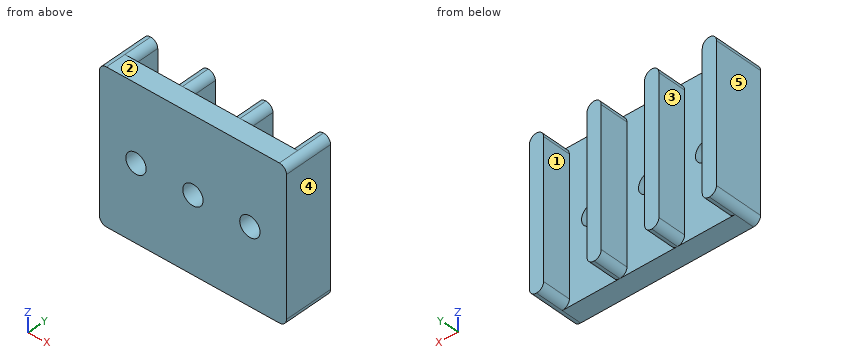
from build123d import *

# Parameters (mm, degrees)
SKETCH1_W           = 46
SKETCH1_H           = 37
SKETCH1_R           = 2.5
BOSS_EXTRUDE1_DEPTH = 12
CUT_EXTRUDE1_START  = -7
SKETCH2_W           = 10.6666
SKETCH2_H           = 37
SKETCH2_R           = 2.5
CUT_EXTRUDE1_DEPTH  = 7
FILLET1_R           = 1.75


with BuildPart() as part:
    # Sketch1 → Boss-Extrude1 (new body)
    with BuildSketch(Plane(origin=(0, 0, 0), x_dir=(1, 0, 0), z_dir=(0, 1, 0))):
        with Locations((-1.399026764, 3.604622871)):
            Rectangle(SKETCH1_W, SKETCH1_H)
        with Locations(Location((-1.399026764, 3.604622871, 0), (0, 0, 270))):
            Circle(SKETCH1_R, mode=Mode.SUBTRACT)
        with Locations(Location((-15.399026764, 3.604622871, 0), (0, 0, 270))):
            Circle(SKETCH1_R, mode=Mode.SUBTRACT)
        with Locations(Location((12.600973236, 3.604622871, 0), (0, 0, 270))):
            Circle(SKETCH1_R, mode=Mode.SUBTRACT)
    extrude(amount=BOSS_EXTRUDE1_DEPTH)

    # Sketch2 → Cut-Extrude1 (cut)
    # profile 1 of 3: a face of its own
    with BuildSketch(Plane(origin=(0, 12, 0), x_dir=(1, 0, 0), z_dir=(0, 1, 0)).offset(CUT_EXTRUDE1_START)):
        with Locations((-15.565726764, 3.604622871)):
            Rectangle(SKETCH2_W, SKETCH2_H)
        with Locations(Location((-15.399026764, 3.604622871, 0), (0, 0, 270))):
            Circle(SKETCH2_R, mode=Mode.SUBTRACT)
    # profile 2 of 3: a face of its own
    with BuildSketch(Plane(origin=(0, 12, 0), x_dir=(1, 0, 0), z_dir=(0, 1, 0)).offset(CUT_EXTRUDE1_START)):
        with Locations((-1.399126764, 3.604622871)):
            Rectangle(SKETCH2_W, SKETCH2_H)
        with Locations(Location((-1.399026764, 3.604622871, 0), (0, 0, 270))):
            Circle(SKETCH2_R, mode=Mode.SUBTRACT)
    # profile 3 of 3: a face of its own
    with BuildSketch(Plane(origin=(0, 12, 0), x_dir=(1, 0, 0), z_dir=(0, 1, 0)).offset(CUT_EXTRUDE1_START)):
        with Locations((12.767473236, 3.604622871)):
            Rectangle(SKETCH2_W, SKETCH2_H)
        with Locations(Location((12.600973236, 3.604622871, 0), (0, 0, 270))):
            Circle(SKETCH2_R, mode=Mode.SUBTRACT)
    extrude(amount=CUT_EXTRUDE1_DEPTH, mode=Mode.SUBTRACT)

    # Fillet1
    fillet1_edges = [part.edges().sort_by_distance(p)[0] for p in [
        (-10.232426764, 8.5, -22.104622871),
        (-10.232426764, 8.5, 14.895377129),
        (-20.899026764, 8.5, 14.895377129),
        (-20.899026764, 8.5, -22.104622871),
        (3.934173236, 8.5, -22.104622871),
        (3.934173236, 8.5, 14.895377129),
        (-6.732426764, 8.5, 14.895377129),
        (-6.732426764, 8.5, -22.104622871),
        (18.100773236, 8.5, -22.104622871),
        (18.100773236, 8.5, 14.895377129),
        (7.434173236, 8.5, 14.895377129),
        (7.434173236, 8.5, -22.104622871),
        (21.600973236, 6, 14.895377129),
        (-24.399026764, 6, 14.895377129),
        (-24.399026764, 6, -22.104622871),
        (21.600973236, 6, -22.104622871),
    ]]
    fillet(fillet1_edges, radius=FILLET1_R - 0.0001)  # a hair under: the kernel refuses the full size


solid = part.part
Could you check a few things on this model? Use its own coordinates, in mm. Face numbers are marked on the shaded views. A direction names the side the tool comes from. Round coordinates to 2 decimals unless told otherwise and drop trailing zeros. Write each loop counter-clockwise with the first axis right and the second up, starting at its lowest first coordinate (ties: lowest second). Pieces come first, ordered by that corner, then holes. Notation, with made-up numbers: (8.25, 34.5) - (41.25, 34.5) arc R22 cw to (41.25, 46.5) - close; hole circle Ø4 at (32.5, 87). An arc over 180 degrees is marked (long way). Put each result on its own line as item: value. Start each with the question number.
(1) For the marked faces 1 and 2, which set-ups out of +Z, -Z, +X, -X, +Y, -Y let a thin tool reach every point of the face, with its end or its side?
(2) I want a section at C-C, the plane z = -13.5. Please give me the cut outline in (x, y), plus the area to 3 significant figures.
(3) Will this pin go through, and if not, where does the flat tip stop? pin 1 (7 mm diameter, centred on x = 12.5, z = -4, fed in from +Y).
(4) I need wall thicknesses on probe 1 along X at (y, z) = (6, 8.5); probe 2 along Y at (x, z) = (-2.5, -8.5); probe 3 along X at (y, z) = (1.25, -5). Which ranges of each line are inside material? Lowest first, please.
(5) Thinking about a two-plate mould opening in X: for the marked faces 3, 4 and 5, which applies, released by +X, released by -X, zero draft, split by the parting line, or undercut?
(6) I want a section at D-D, the plane y = 4. Please give me the cut outline in (x, z), plus the area to 3 significant figures.
(7) I want a section at B-B, the plane x = 11. Please give me the cut outline in (y, z).
(8) I want a section at A-A, the plane y = 6.5. Give the number of separate pieces and of enclosed holes in the cut face, plus the area to 3 significant figures.
Here are the results:
1. face 1: +Z, -Z, +Y
1. face 2: +Z, +X, -X, +Y, -Y
2. outline: (-24.4, 0) - (21.6, 0) - (21.6, 12) - (18.1, 12) - (18.1, 5) - (7.43, 5) - (7.43, 12) - (3.93, 12) - (3.93, 5) - (-6.73, 5) - (-6.73, 12) - (-10.23, 12) - (-10.23, 5) - (-20.9, 5) - (-20.9, 12) - (-24.4, 12) - close
2. area: 328 mm^2
3. pin 1: stops at y = 5
4. probe 1: x = -24.4 to -20.9, -10.23 to -6.73, 3.93 to 7.43, 18.1 to 21.6
4. probe 2: y = 0 to 5
4. probe 3: x = -24.4 to -17.47, -13.32 to -3.47, 0.68 to 10.53, 14.68 to 21.6
5. face 3: undercut
5. face 4: released by +X
5. face 5: released by -X
6. outline: (-24.4, -20.35) arc R1.75 ccw to (-22.65, -22.1) - (19.85, -22.1) arc R1.75 ccw to (21.6, -20.35) - (21.6, 13.15) arc R1.75 ccw to (19.85, 14.9) - (-22.65, 14.9) arc R1.75 ccw to (-24.4, 13.15) - close; hole circle Ø5 at (-15.4, -3.6); hole circle Ø5 at (-1.4, -3.6); hole circle Ø5 at (12.6, -3.6)
6. area: 1,640 mm^2
7. outline: (0, -22.1) - (5, -22.1) - (5, -5.52) - (0, -5.52) - close; (0, -1.68) - (5, -1.68) - (5, 14.9) - (0, 14.9) - close
8. separate pieces: 4
8. enclosed holes: 0
8. area: 507 mm^2
